Geometry check sheet. Reference: the model listing, model coordinates, mm. Face numbers are marked on the shaded views. A direction names the side the tool comes from. Coordinates: 2 decimals unless noted, no trailing zeros. Order: outer loops, then holes, each group sorted by start corner. A loop starts at its lowest first (then second) coordinate and runs counter-clockwise, first axis right, second up.
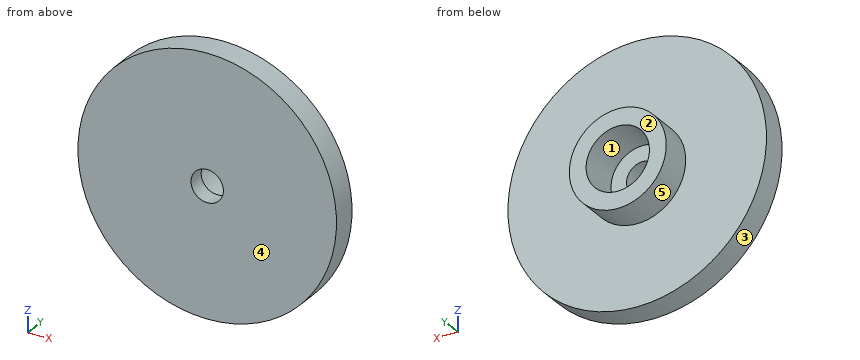
```python
from build123d import *

# Parameters (mm, degrees)
SKETCH_1_R          = 10
SKETCH_1_R_2        = 1.25
EXTRUDE_1_DEPTH     = 2
SKETCH_2_R          = 3.75
EXTRUDE_2_DEPTH     = 2.5
SKETCH_4_R          = 2.45
CUT_EXTRUDE_1_DEPTH = 3.2


with BuildPart() as part:
    # 草图1 → 凸台-拉伸1 (new body)
    with BuildSketch(Plane(origin=(0, 0, 0), x_dir=(1, 0, 0), z_dir=(0, 1, 0))):
        with Locations(Location((0, 0, 0), (0, 0, 270))):
            Circle(SKETCH_1_R)
        with Locations(Location((0, 0, 0), (0, 0, 270))):
            Circle(SKETCH_1_R_2, mode=Mode.SUBTRACT)
    extrude(amount=EXTRUDE_1_DEPTH)

    # 草图2 → 凸台-拉伸2 (add)
    with BuildSketch(Plane(origin=(0, 2, 0), x_dir=(1, 0, 0), z_dir=(0, 1, 0))):
        with Locations(Location((0, 0, 0), (0, 0, 270))):
            Circle(SKETCH_2_R)
    extrude(amount=EXTRUDE_2_DEPTH)

    # 草图4 → 切除-拉伸1 (cut)
    with BuildSketch(Plane(origin=(0, 4.5, 0), x_dir=(1, 0, 0), z_dir=(0, 1, 0))):
        with Locations(Location((0, 0, 0), (0, 0, 270))):
            Circle(SKETCH_4_R)
    extrude(amount=-CUT_EXTRUDE_1_DEPTH, mode=Mode.SUBTRACT)


solid = part.part
```
Item 1: Depth check by flat-ended pin: P1, Ø1, axis at x = 4.5, y = 0.5, coming from the -Z side; P2, Ø1, axis at y = 1.5, z = -5, coming from the -X side; P3, Ø1, axis at y = 0.5, z = -8, coming from the +X side. Enter the tip coordinate at first touch or a pass-through.
Item 2: Sectioned sample at A-A (x = 0). Record the cut outline in (y, z).
Item 3: Tool access check on the marked faces 4 and 5. Record the directions out of +Z, -Z, +X, -X, +Y, -Y that give a thin tool (end or side, any length) a straight path to the whole face; none if there is none.
Item 4: Release check for a two-part mould opening along Z. For the marked faces 1, 2 and 3 record: pulls with the +Z half, pulls with the -Z half, needs draft (parallel to the pull), parting line crosses it, or undercut.
Item 5: Thickness scan on line 1 along Y through (x, z) = (6.5, -2.75); line 2 along X through (y, z) = (0.3, 0); line 3 along Y through (x, z) = (-1.5, -1.5). Record the ranges inside material, lowest first.
Item 6: Sectioned sample at B-B (z = 0). Record the cut outline in (x, y).
Item 7: Sectioned sample at D-D (x = 2). Record the cut outline in (y, z), and give its area (3 significant figures).
Item 8: Sectioned sample at C-C (y = 4.25). Record the cut outline in (x, z).
Geometry check:
1. P1: stops at z = -9.17
1. P2: stops at x = -8.93
1. P3: stops at x = 6.61
2. outline: (0, -10) - (2, -10) - (2, -3.75) - (4.5, -3.75) - (4.5, -2.45) - (1.3, -2.45) - (1.3, -1.25) - (0, -1.25) - close; (0, 1.25) - (1.3, 1.25) - (1.3, 2.45) - (4.5, 2.45) - (4.5, 3.75) - (2, 3.75) - (2, 10) - (0, 10) - close
3. face 4: +Z, -Z, +X, -X, -Y
3. face 5: +Y
4. face 1: undercut
4. face 2: needs draft
4. face 3: parting line crosses it
5. line 1: y = 0 to 2
5. line 2: x = -10 to -1.25, 1.25 to 10
5. line 3: y = 0 to 1.3
6. outline: (-10, 0) - (-1.25, 0) - (-1.25, 1.3) - (-2.45, 1.3) - (-2.45, 4.5) - (-3.75, 4.5) - (-3.75, 2) - (-10, 2) - close; (1.25, 0) - (10, 0) - (10, 2) - (3.75, 2) - (3.75, 4.5) - (2.45, 4.5) - (2.45, 1.3) - (1.25, 1.3) - close
7. outline: (0, -9.8) - (2, -9.8) - (2, -3.17) - (4.5, -3.17) - (4.5, -1.42) - (1.3, -1.42) - (1.3, 1.42) - (4.5, 1.42) - (4.5, 3.17) - (2, 3.17) - (2, 9.8) - (0, 9.8) - close
7. area: 46.0 mm2
8. outline: circle Ø7.5 at (0, 0); hole circle Ø4.9 at (0, 0)
